Could you check a few things on this drawing? It's one solid part, dimensions in mm from its lowest x, y, z. Give positions to 0.01 mm unless a question says otherwise; leave off trailing zeros. Loops run counter-clockwise (first coordinate to the right, second up) from the corner with the lowest first, then second, coordinate; pieces in that order, holes last.
Q1. I need wall thicknesses on probe 1 along Z at (x, y) = (10, 0.6); probe 2 along X at (y, z) = (0.95, 7.75); probe 3 along Z at (x, y) = (8, 1.6). Which ranges of each line are inside material? Lowest first, please.
Q2. Suppose I cut it at B-B (y = 4.15). List the corners of the cut face in (x, z) for me.
Q3. Suppose I cut it at A-A (x = 10). List the corners of the cut face in (y, z) for me.
Q4. Suppose I cut it at C-C (x = 18.5). List the corners of the cut face in (y, z) for me.
Q5. I'm going to push a flat-ended pin straight in: P1, Ø1.5, axis at x = 9.5, y = 3.5, coming from the -Z side. Where does the tip first touch, or does it pass through?
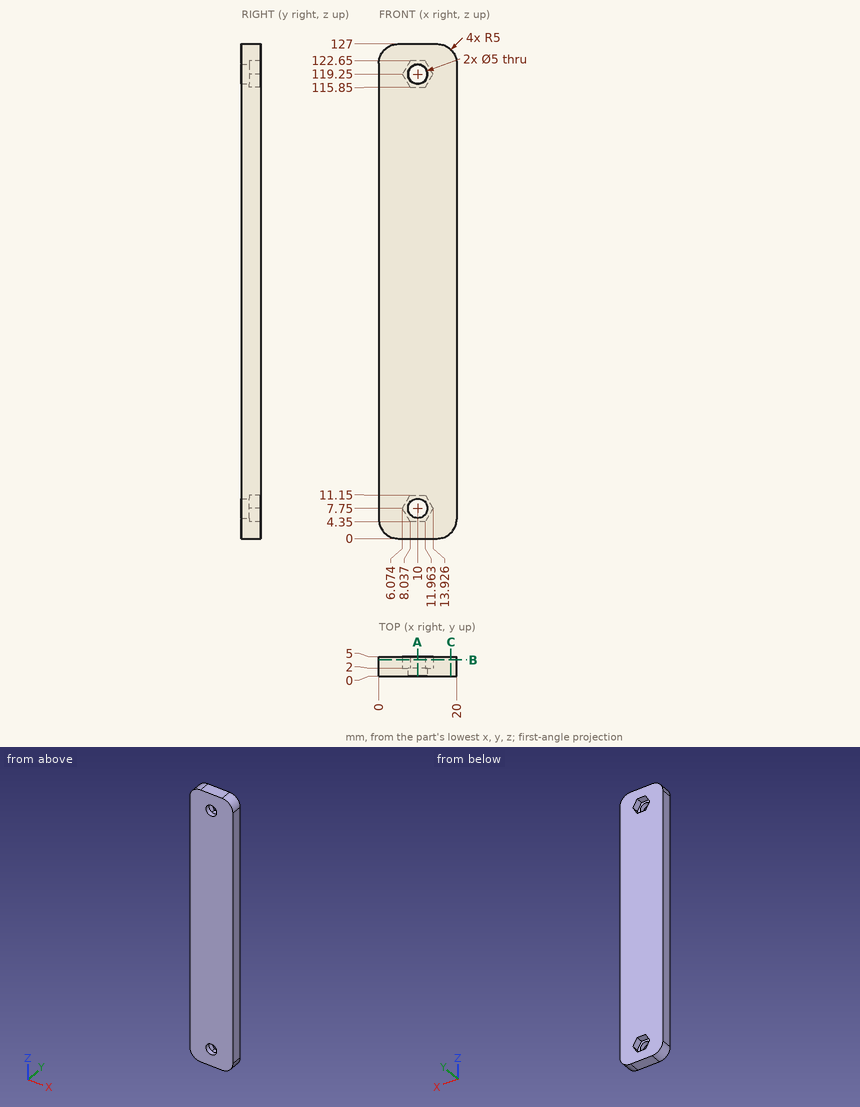
Solutions:
1. probe 1: z = 0 to 5.25, 10.25 to 116.75, 121.75 to 127
1. probe 2: x = 0 to 7.5, 12.5 to 20
1. probe 3: z = 0 to 6.25, 9.25 to 117.75, 120.75 to 127
2. outline: (0, 5) arc R5 ccw to (5, 0) - (15, 0) arc R5 ccw to (20, 5) - (20, 122) arc R5 ccw to (15, 127) - (5, 127) arc R5 ccw to (0, 122) - close; hole (6.07, 7.75) - (8.04, 4.35) - (11.96, 4.35) - (13.93, 7.75) - (11.96, 11.15) - (8.04, 11.15) - close; hole (6.07, 119.25) - (8.04, 115.85) - (11.96, 115.85) - (13.93, 119.25) - (11.96, 122.65) - (8.04, 122.65) - close
3. outline: (0, 0) - (5, 0) - (5, 4.35) - (2, 4.35) - (2, 5.25) - (0, 5.25) - close; (0, 10.25) - (2, 10.25) - (2, 11.15) - (5, 11.15) - (5, 115.85) - (2, 115.85) - (2, 116.75) - (0, 116.75) - close; (0, 121.75) - (2, 121.75) - (2, 122.65) - (5, 122.65) - (5, 127) - (0, 127) - close
4. outline: (0, 1.43) - (5, 1.43) - (5, 125.57) - (0, 125.57) - close
5. P1: stops at z = 0
